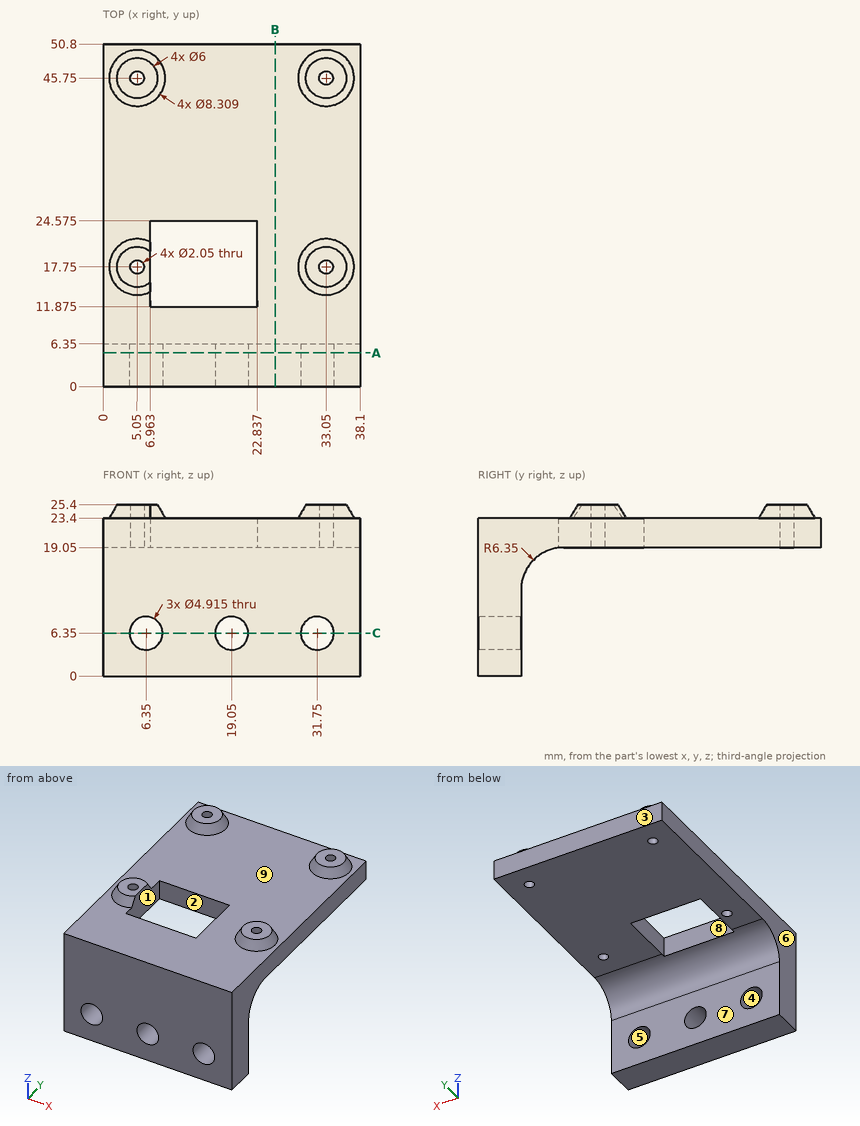
Job drawing, mm, ordinate dimensions from the low corner. One solid piece. A direction names the side the tool comes from. Give positions to 0.01 mm unless a question says otherwise; leave off trailing zeros. Loops run counter-clockwise (first coordinate to the right, second up) from the corner with the lowest first, then second, coordinate; pieces in that order, holes last. Notation, with made-up numbers: (24.5, 57) - (83.5, 57) arc R17 ccw to (83.5, 80) - close; hole circle Ø5 at (-31, 86). An arc over 180 degrees is marked (long way). Use one line per item in the form item = value.
(1) Drop flat-ended pins along their axis: P1, Ø4, axis at y = 42, z = 16, coming from the -X side; P2, Ø6.5, axis at x = 25, z = 7.5, coming from the +Y side; P3, Ø3.5, axis at x = 5.05, y = 45.75, coming from the +Z side; P4, Ø2.5, axis at x = 33.05, y = 45.75, coming from the -Z side. Give the stop position or say it passes through.
Determined:
P1 = through
P2 = 6.35
P3 = 25.4
P4 = 19.05
(2) Drill centre lines: L1, parallel to Y at x = 5.05, z = 21 (1 decimal); L2, parallel to X at y = 3.5, z = 6.35; L3, parallel to Y at x = 16, z = 19.5 (1 decimal). Where is each one in solid material? Low to high.
Determined:
L1 = 0 to 16.7, 18.8 to 44.7, 46.8 to 50.8
L2 = 0 to 3.89, 8.81 to 16.59, 21.51 to 29.29, 34.21 to 38.1
L3 = 0 to 11.9, 24.6 to 50.8
(3) Cut at C-C (z = 6.35). Give the cut face in (x, y), then the cut area to 3 significant figures.
Determined:
outline = (0, 0) - (3.89, 0) - (3.89, 6.35) - (0, 6.35) - close; (8.81, 0) - (16.59, 0) - (16.59, 6.35) - (8.81, 6.35) - close; (21.51, 0) - (29.29, 0) - (29.29, 6.35) - (21.51, 6.35) - close; (34.21, 0) - (38.1, 0) - (38.1, 6.35) - (34.21, 6.35) - close
area = 148 mm^2
(4) Cut at B-B (x = 25.5). Give the cut face in (y, z).
Determined:
outline = (0, 0) - (6.35, 0) - (6.35, 12.7) arc R6.35 cw to (12.7, 19.05) - (50.8, 19.05) - (50.8, 23.4) - (0, 23.4) - close
(5) Pull direction Y, two halves, no side cores. Call the marked faces 1, 2, 3 and 4: pulls with the +Y half, pulls with the -Y half, needs draft (parallel to the pull), parting line crosses it, or undercut.
Determined:
face_1 = undercut
face_2 = undercut
face_3 = pulls with the +Y half
face_4 = needs draft
(6) 3-axis set-ups, long thin cutter, end or side, ignore diameter. For the marked faces 5, 6, 7, 8 and 9: which of +Z, -Z, +X, -X, +Y, -Y reach the whole face in a straight line?
Determined:
face_5 = +Y, -Y
face_6 = +Z, -Z, -X, +Y, -Y
face_7 = -Z, +X, -X, +Y
face_8 = +Z, -Z
face_9 = +Z
(7) Cut at A-A (y = 5). Count the separate pieces of the cut face and the enclosed holes in it.
Determined:
separate_pieces = 1
enclosed_holes = 3
